from build123d import *

# Parameters (mm, degrees)
SKETCH1_R                = 19.05
BASE_EXTRUDE_DEPTH       = 431.8
SKETCH4_R                = 7.62
BOSS_EXTRUDE1_DEPTH      = 6.35
BOSS_EXTRUDE1_DEPTH_BACK = 6.35


with BuildPart() as part:
    # Sketch1 → Base-Extrude (new body)
    with BuildSketch(Plane.XY):
        Circle(SKETCH1_R)
    extrude(amount=-BASE_EXTRUDE_DEPTH)

    # Sketch4 → Boss-Extrude1 (add, two sides)
    with BuildSketch(Plane(origin=(0, 0, 0), x_dir=(-1, 0, 0), z_dir=(0, 1, 0))) as boss_extrude1_sk:
        with BuildLine():
            Line((-18.231166151, -59.074644757), (-18.231166151, 0))
            ThreePointArc((-18.231166151, 0), (-47.768488529, -29.537322378), (-18.231166151, -59.074644757))
        make_face()
        with Locations((-36.011166151, -29.537322378)):
            Circle(SKETCH4_R, mode=Mode.SUBTRACT)
    extrude(amount=BOSS_EXTRUDE1_DEPTH)
    extrude(boss_extrude1_sk.sketch, amount=-BOSS_EXTRUDE1_DEPTH_BACK)


solid = part.part
Here's how the part is built. I have some questions about the finished solid (model axes, mm). A direction names the side the tool comes from. Round coordinates to 2 decimals unless told otherwise and drop trailing zeros. Loops run counter-clockwise (first coordinate to the right, second up) from the corner with the lowest first, then second, coordinate; pieces in that order, holes last. Notation, with made-up numbers: M 5,13.25 L 61,13.25 A27 ccw 61,44.25 Z; hole C 10,88 d9. An arc over 180 degrees is marked long. Write each question's results on one line, items separated by ' | '. Start each with the question number.
(1) On a 3-axis mill with a long thin cutter (end or side, diameter ignored), from which of +Z, -Z, +X, -X, +Y, -Y can I reach the whole of each face in a straight line? I mean faces 1 (the flat face through (27, -6.35, -29)), 2 (the flat face through (0, 0, -431.8)), 3 (the flat face through (27, 6.35, -29)). Say none if no direction works.
(2) I want a section at B-B (x = -9.5). Please give me the cut outline in (y, z).
(3) I want a section at C-C (x = 7). Please give me the cut outline in (y, z).
(4) Will these pins go through, and if not, where does the flat tip stop? P1, Ø23.5, axis at x = 34, z = -43, coming from the +Y side; P2, Ø6, axis at x = -12, z = -69, coming from the +Y side; P3, Ø20, axis at x = 36.01, z = -29.54, coming from the -Y side.
(5) If I drill on probe 1 along Y at (x, z) = (0.5, -353.5); probe 2 along X at (y, z) = (-1, -97); probe 3 along Z at (x, y) = (34.5, -0.5), over which ranges is the centre line in solid material (lowest first)? Write a range as from..to.
(6) I want a section at A-A (z = -383.5). Please give me the cut outline in (x, y), then the cut area to 3 significant figures.
Solved:
1) face 1: +Z, -Z, +X, -Y | face 2: -Z, +X, -X, +Y, -Y | face 3: +Z, -Z, +X, +Y
2) outline: M -16.51,-431.8 L 16.51,-431.8 L 16.51,0 L -16.51,0 Z
3) outline: M -17.72,-431.8 L 17.72,-431.8 L 17.72,0 L -17.72,0 Z
4) P1: stops at y = 6.35 | P2: stops at y = 16.79 | P3: stops at y = -6.35
5) probe 1: y = -19.04..19.04 | probe 2: x = -19.02..19.02 | probe 3: z = -54.19..-37.01, -22.07..-4.88
6) outline: C 0,0 d38.1 | area: 1,140 mm²
